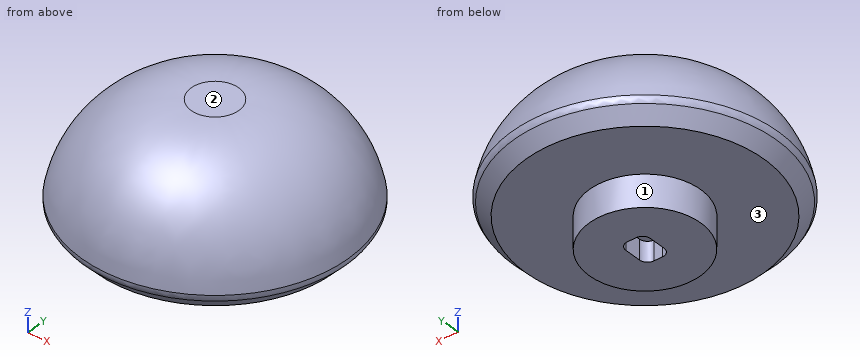
Autodesk Fusion 360 part; units mm, degrees
sketch "Sketch1" plane through (0, 0, 0) normal (0, 1, 0) x (1, 0, 0)
  line L0 (0, 0) -> (7, 0)
  line L1 (7, 0) -> (7, -4)
  line L2 (7, -4) -> (17, -4)
  line L3 (0, -18) -> (0, 0)
  line L4 (0, -18) -> (3, -18)
  arc A0 (3, -18) -> (17, -4) centre (3, -4) ccw
  dimension "d1" = 7
  dimension "d2" = 4
  dimension "d3" = 10
  dimension "d4" = 3
  dimension "d5" = 18
revolve "Revolve1" add sketch "Sketch1" angle 360 about axis through (0, 0, 18) along (0, 0, -1)
sketch "Sketch2" plane through (0, 0, 0) normal (0, 0, -1) x (1, 0, 0)
  circle A0 centre (0, 0) radius 7
  line L0 (1.55, 1.05) -> (1.55, -1.05)
  line L1 (-1.55, 1.05) -> (-1.55, -1.05)
  line L2 (0.55, -2.05) -> (-0.55, -2.05)
  line L3 (0.55, 2.05) -> (-0.55, 2.05)
  arc A1 (0.55, -2.05) -> (1.55, -1.05) centre (0.55, -1.05) ccw
  arc A2 (-0.55, 2.05) -> (-1.55, 1.05) centre (-0.55, 1.05) ccw
  arc A3 (-1.55, -1.05) -> (-0.55, -2.05) centre (-0.55, -1.05) ccw
  arc A4 (1.55, 1.05) -> (0.55, 2.05) centre (0.55, 1.05) ccw
  point P0 (0, -2.05)
  point P1 (1.55, 2.05)
  point P2 (1.55, -2.05)
  point P3 (1.55, 0)
  point P4 (-1.55, 2.05)
  dimension "d11" = 4.1
  dimension "d12" = 3.1
  dimension "d13" = 1
extrude "Extrude1" cut sketch "Sketch2" against normal blind 2.5 contours L0 L1 L2 L3 A1 A2 A3 A4
chamfer "Chamfer1" distance 2 angle 45 1 edges at (-15.8496, -6.1475, 4)
fillet "Fillet1" radius 1 1 edges at (15.7164, -6.0958, 5.9949)
Geometry: final body of the model. Coordinates: model frame, mm. Face numbers are marked on the shaded views. Round coordinates to 2 decimals unless told otherwise and drop trailing zeros. Write each question's results on one line, items separated by ' | '. Start each with the question number.
1) First-contact query: P1, Ø3, axis at x = -2, z = 8.5, coming from the +Y side; P2, Ø5, axis at x = 7.5, z = 9, coming from the +Y side; P3, Ø0.6, axis at y = 0, z = 1, coming from the +X side. Flat tips, straight axial feed; report the tip coordinate or a pass-through.
2) Line query: probe 1 along Z at (x, y) = (0.5, -1); probe 2 along Z at (x, y) = (3.5, 0); probe 3 along Y at (x, z) = (-11, 5.75). Output: solid intervals per line, ascending. Write a range as [from, to].
3) Mould query, pull axis Z, two halves, no side actions, for the marked faces 1, 2 and 3. Classes: released by +Z, released by -Z, zero draft, split by the parting line, or undercut.
Verdict:
1) P1: stops at y = 16.59 | P2: stops at y = 15.62 | P3: stops at x = 7
2) probe 1: z = [2.5, 18] | probe 2: z = [0, 17.99] | probe 3: y = [-12.45, 12.45]
3) face 1: zero draft | face 2: released by +Z | face 3: released by -Z
